The model under review builds one solid part; all positions refer to its coordinate system, in mm. Face numbers are marked on the shaded views. A direction names the side the tool comes from. Give positions to 0.01 mm unless a question says otherwise; leave off trailing zeros. Order: outer loops, then holes, each group sorted by start corner. A loop starts at its lowest first (then second) coordinate and runs counter-clockwise, first axis right, second up.
```python
from build123d import *

# Parameters (mm, degrees)
SKETCH2_W              = 101.6
SKETCH2_H              = 114.3
BOSS_EXTRUDE1_DEPTH    = 63.5
SKETCH4_W              = 101.6
SKETCH4_H              = 5.5
CUT_EXTRUDE2_DEPTH     = 141.276084918
SKETCH6_W              = 101.6
SKETCH6_H              = 3
CUT_EXTRUDE4_DEPTH     = 108.56226104
SKETCH3_R              = 18
CUT_EXTRUDE1_DEPTH     = 106.492369392
SKETCH5_R              = 23.5
CUT_EXTRUDE3_DEPTH     = 46.24
M8_TAPPED_HOLE1_D      = 6.8
M8_TAPPED_HOLE1_DEPTH  = 26.35
M8_TAPPED_HOLE1_TIP    = 2.042926105
CHAMFER1_SIZE          = 1
CHAMFER1_SIZE2         = 0.577350269
CUT_EXTRUDE6_START     = -48.5
SKETCH9_R              = 19
CUT_EXTRUDE6_DEPTH     = 1.6
CUT_EXTRUDE7_DEPTH     = 5.08
M12_TAPPED_HOLE1_D     = 10.2
M12_TAPPED_HOLE1_DEPTH = 32.75
M12_TAPPED_HOLE1_TIP   = 3.064389157
SKETCH14_W             = 4.8
SKETCH14_H             = 111.3
CUT_EXTRUDE8_DEPTH     = 106.492369392
FILLET1_R              = 0.79375
CUT_EXTRUDE9_START     = 1.2954
SKETCH15_R             = 24.008
SKETCH15_R_2           = 23.5
CUT_EXTRUDE9_DEPTH     = 1.2954


with BuildPart() as part:
    # Sketch2 → Boss-Extrude1 (new body)
    with BuildSketch(Plane.XY):
        with Locations((0, -17.85)):
            Rectangle(SKETCH2_W, SKETCH2_H)
    extrude(amount=BOSS_EXTRUDE1_DEPTH)

    # Sketch4 → Cut-Extrude2 (cut, through all)
    with BuildSketch(Plane(origin=(0, 39.3, 0), x_dir=(1, 0, 0), z_dir=(0, 1, 0))):
        with Locations((0, -60.75)):
            Rectangle(SKETCH4_W, SKETCH4_H)
    extrude(amount=-CUT_EXTRUDE2_DEPTH, mode=Mode.SUBTRACT)

    # Sketch6 → Cut-Extrude4 (cut, through all)
    with BuildSketch(Plane.XY.offset(58)):
        with Locations((0, -73.5)):
            Rectangle(SKETCH6_W, SKETCH6_H)
    extrude(amount=-CUT_EXTRUDE4_DEPTH, mode=Mode.SUBTRACT)

    # Sketch3 → Cut-Extrude1 (cut, through all)
    with BuildSketch(Plane.XY.offset(58)):
        Circle(SKETCH3_R)
    extrude(amount=-CUT_EXTRUDE1_DEPTH, mode=Mode.SUBTRACT)

    # Sketch5 → Cut-Extrude3 (cut)
    with BuildSketch(Plane.XY.offset(58)):
        Circle(SKETCH5_R)
    extrude(amount=-CUT_EXTRUDE3_DEPTH, mode=Mode.SUBTRACT)

    # M8 Tapped Hole1
    with Locations(Plane.XY.offset(58)):
        with Locations((0, 29.25), (25.331243061, 14.625), (25.331243061, -14.625), (0, -29.25), (-25.331243061, -14.625), (-25.331243061, 14.625)):
            Hole(M8_TAPPED_HOLE1_D / 2, depth=M8_TAPPED_HOLE1_DEPTH)
            with Locations((0, 0, -(M8_TAPPED_HOLE1_DEPTH + M8_TAPPED_HOLE1_TIP / 2))):  # 118° drill point
                Cone(0, M8_TAPPED_HOLE1_D / 2, M8_TAPPED_HOLE1_TIP, mode=Mode.SUBTRACT)

    # Chamfer1
    chamfer1_edges = [part.edges().sort_by_distance(p)[0] for p in [
        (-23.5, 0, 58),
    ]]
    chamfer1_side = [part.faces().sort_by_distance(p)[0] for p in [
        (-23.5, 0, 34.88),
    ]]
    chamfer(chamfer1_edges, length=CHAMFER1_SIZE, length2=CHAMFER1_SIZE2, reference=chamfer1_side[0])

    # Sketch9 → Cut-Extrude6 (cut)
    with BuildSketch(Plane.XY.offset(58).offset(CUT_EXTRUDE6_START)):
        Circle(SKETCH9_R)
    extrude(amount=-CUT_EXTRUDE6_DEPTH, mode=Mode.SUBTRACT)

    # Sketch10 → Cut-Extrude7 (cut)
    with BuildSketch(Plane.XZ.offset(72)):
        with BuildLine():
            Line((-25.4, 36), (25.4, 36))
            ThreePointArc((25.4, 36), (31.4, 30), (25.4, 24))
            Line((25.4, 24), (-25.4, 24))
            ThreePointArc((-25.4, 24), (-31.4, 30), (-25.4, 36))
        make_face()
    extrude(amount=-CUT_EXTRUDE7_DEPTH, mode=Mode.SUBTRACT)

    # M12 Tapped Hole1
    with Locations(Plane(origin=(0, -72, 0), x_dir=(-1, 0, 0), z_dir=(0, -1, 0))):
        with Locations((31, -46), (-31, -46), (-31, -14), (31, -14)):
            Hole(M12_TAPPED_HOLE1_D / 2, depth=M12_TAPPED_HOLE1_DEPTH)
            with Locations((0, 0, -(M12_TAPPED_HOLE1_DEPTH + M12_TAPPED_HOLE1_TIP / 2))):  # 118° drill point
                Cone(0, M12_TAPPED_HOLE1_D / 2, M12_TAPPED_HOLE1_TIP, mode=Mode.SUBTRACT)

    # Sketch14 → Cut-Extrude8 (cut, through all)
    with BuildSketch(Plane(origin=(0, 0, 0), x_dir=(-1, 0, 0), z_dir=(0, 0, -1))):
        with Locations((-48.4, -16.35)):
            Rectangle(SKETCH14_W, SKETCH14_H)
        with Locations((48.4, -16.35)):
            Rectangle(SKETCH14_W, SKETCH14_H)
    extrude(amount=-CUT_EXTRUDE8_DEPTH, mode=Mode.SUBTRACT)

    # Fillet1
    fillet1_edges = [part.edges().sort_by_distance(p)[0] for p in [
        (-31.4, -66.92, 30),
        (0, -66.92, 36),
        (31.4, -66.92, 30),
        (0, -66.92, 24),
    ]]
    fillet(fillet1_edges, radius=FILLET1_R)

    # Sketch15 → Cut-Extrude9 (cut)
    with BuildSketch(Plane.XY.offset(11.76).offset(CUT_EXTRUDE9_START)):
        Circle(SKETCH15_R)
        Circle(SKETCH15_R_2, mode=Mode.SUBTRACT)
    extrude(amount=-CUT_EXTRUDE9_DEPTH, mode=Mode.SUBTRACT)


solid = part.part
```
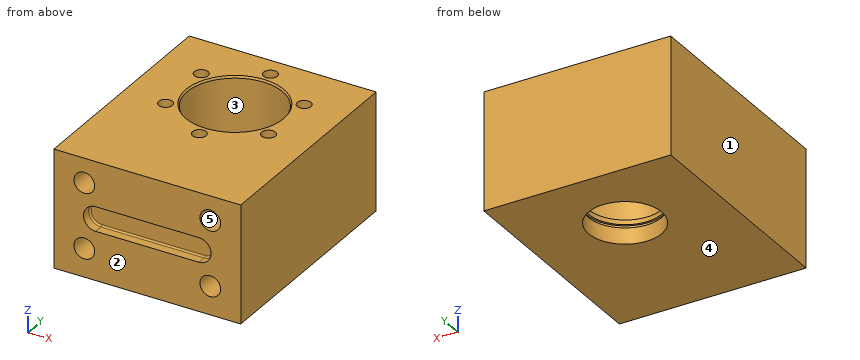
Item 1: For the marked faces 4 and 5, list the 3-axis set-ups (+Z, -Z, +X, -X, +Y, -Y) from which the entire face can be reached by the end or side of a thin tool; tool diameter is ignored.
Values found:
face 4: -Z, +X, -X, +Y, -Y
face 5: -Y
Item 2: Draft analysis for pull direction Y (two halves, no side actions). For the marked faces 1, 2 and 3, state which applies: released by +Y, released by -Y, zero draft, split by the parting line, or undercut.
Values found:
face 1: zero draft
face 2: released by -Y
face 3: undercut
Item 3: For line 1 (Y direction, x = 0, z = 42); line 2 (X direction, y = -62, z = 46); line 3 (Z direction, x = 31, y = -52.5), list the stretches that pass through material, from the lowest coordinate up.
Values found:
line 1: y = -72 to -32.65, -25.85 to -23.5, 23.5 to 25.85, 32.65 to 39.3
line 2: x = -46 to -36.1, -25.9 to 25.9, 36.1 to 46
line 3: z = 0 to 8.9, 19.1 to 40.9, 51.1 to 58
Item 4: Clearance check with flat-ended pins moving along their axes: pin 1 Ø5.5 at (x, y) = (25.33, 14.62) entering from +Z; pin 2 Ø3 at (x, z) = (1.5, 29) entering from -Y; pin 3 Ø14.5 at (x, y) = (11, -8) entering from +Z. State where each tip first meets the part, or that it passes through.
Values found:
pin 1: stops at z = 31.26
pin 2: stops at y = -66.92
pin 3: stops at z = 11.76
Item 5: Take a section at A-A (y = -48). Give the boundary of the cut face in (x, z), and give its area (3 significant figures).
Values found:
outline: (-46, 0) - (46, 0) - (46, 58) - (-46, 58) - close; hole circle Ø10.2 at (-31, 14); hole circle Ø10.2 at (-31, 46); hole circle Ø10.2 at (31, 14); hole circle Ø10.2 at (31, 46)
area: 5,010 mm2
Item 6: Take a section at B-B (z = 6.5). Give the boundary of the cut face in (x, y).
Values found:
outline: (-46, -72) - (46, -72) - (46, 39.3) - (-46, 39.3) - close; hole circle Ø36 at (0, 0)
Item 7: Take a section at C-C (y = 0). Give the boundary of the cut face in (x, z).
Values found:
outline: (-46, 0) - (-18, 0) - (-18, 7.9) - (-19, 7.9) - (-19, 9.5) - (-18, 9.5) - (-18, 11.76) - (-24.01, 11.76) - (-24.01, 13.06) - (-23.5, 13.06) - (-23.5, 57) - (-24.08, 58) - (-46, 58) - close; (18, 0) - (46, 0) - (46, 58) - (24.08, 58) - (23.5, 57) - (23.5, 13.06) - (24.01, 13.06) - (24.01, 11.76) - (18, 11.76) - (18, 9.5) - (19, 9.5) - (19, 7.9) - (18, 7.9) - close
